Geometry: final body of the model. Coordinates: model frame, mm. A direction names the side the tool comes from. Give positions to 0.01 mm unless a question says otherwise; leave off trailing zeros. Loops run counter-clockwise (first coordinate to the right, second up) from the corner with the lowest first, then second, coordinate; pieces in that order, holes last. Notation, with made-up numbers: (27.5, -9.5) - (79.5, -9.5) arc R19 cw to (79.5, 13.5) - close; hole circle Ø11 at (-15.75, -33.75). An arc over 180 degrees is marked (long way). Answer in a Markdown table with one row per item.
from build123d import *

# Parameters (mm, degrees)
SKETCH1_W           = 114.3
SKETCH1_H           = 177.8
BOSS_EXTRUDE1_DEPTH = 3.9624
CUT_EXTRUDE2_START  = 3.9624
SKETCH2_W           = 184.15
SKETCH2_H           = 53.975
CUT_EXTRUDE2_DEPTH  = 110.721716912
CUT_EXTRUDE4_START  = 3.9624
SKETCH3_R           = 5.1562
CUT_EXTRUDE4_DEPTH  = 110.721716912
CUT_EXTRUDE6_START  = 3.9624
SKETCH4_R           = 5.1562
CUT_EXTRUDE6_DEPTH  = 110.721716912
CUT_EXTRUDE8_START  = 3.9624
SKETCH5_R           = 5.1562
CUT_EXTRUDE8_DEPTH  = 110.721716912
CUT_EXTRUDE10_START = 3.9624
SKETCH6_R           = 2.5781
CUT_EXTRUDE10_DEPTH = 114.3
CUT_EXTRUDE12_START = 3.9624
SKETCH7_R           = 2.5781
CUT_EXTRUDE12_DEPTH = 114.3


with BuildPart() as part:
    # Sketch1 → Boss-Extrude1 (new, symmetric)
    with BuildSketch(Plane(origin=(0, 0, 0), x_dir=(1, 0, 0), z_dir=(0, 1, 0))):
        Rectangle(SKETCH1_W, SKETCH1_H)
    extrude(amount=BOSS_EXTRUDE1_DEPTH, both=True)

    # Sketch2 → Cut-Extrude2 (cut, through all)
    with BuildSketch(Plane(origin=(0, 0, 0), x_dir=(1, 0, 0), z_dir=(0, 1, 0)).offset(CUT_EXTRUDE2_START)):
        with Locations((-79.375, -7.9375)):
            Rectangle(SKETCH2_W, SKETCH2_H)
    extrude(amount=-CUT_EXTRUDE2_DEPTH, mode=Mode.SUBTRACT)

    # Sketch3 → Cut-Extrude4 (cut, through all)
    with BuildSketch(Plane(origin=(0, 0, 0), x_dir=(1, 0, 0), z_dir=(0, 1, 0)).offset(CUT_EXTRUDE4_START)):
        with Locations(Location((-38.1, -79.375, 0), (0, 0, 270))):
            Circle(SKETCH3_R)
        with Locations(Location((-38.1, 79.375, 0), (0, 0, 270))):
            Circle(SKETCH3_R)
    extrude(amount=-CUT_EXTRUDE4_DEPTH, mode=Mode.SUBTRACT)

    # Sketch4 → Cut-Extrude6 (cut, through all)
    with BuildSketch(Plane(origin=(0, 0, 0), x_dir=(1, 0, 0), z_dir=(0, 1, 0)).offset(CUT_EXTRUDE6_START)):
        with Locations(Location((1.5748, -79.375, 0), (0, 0, 270))):
            Circle(SKETCH4_R)
        with Locations(Location((1.5748, 79.375, 0), (0, 0, 270))):
            Circle(SKETCH4_R)
    extrude(amount=-CUT_EXTRUDE6_DEPTH, mode=Mode.SUBTRACT)

    # Sketch5 → Cut-Extrude8 (cut, through all)
    with BuildSketch(Plane(origin=(0, 0, 0), x_dir=(1, 0, 0), z_dir=(0, 1, 0)).offset(CUT_EXTRUDE8_START)):
        with Locations(Location((41.275, -79.375, 0), (0, 0, 270))):
            Circle(SKETCH5_R)
        with Locations(Location((41.275, 79.375, 0), (0, 0, 270))):
            Circle(SKETCH5_R)
    extrude(amount=-CUT_EXTRUDE8_DEPTH, mode=Mode.SUBTRACT)

    # Sketch6 → Cut-Extrude10 (cut)
    with BuildSketch(Plane(origin=(0, 0, 0), x_dir=(1, 0, 0), z_dir=(0, 1, 0)).offset(CUT_EXTRUDE10_START)):
        with Locations(Location((-41.9862, -45.5422, 0), (0, 0, 270))):
            Circle(SKETCH6_R)
        with Locations(Location((-7.0612, -45.5422, 0), (0, 0, 270))):
            Circle(SKETCH6_R)
        with Locations(Location((27.8638, -45.5422, 0), (0, 0, 270))):
            Circle(SKETCH6_R)
        with Locations(Location((-41.9862, 28.8798, 0), (0, 0, 270))):
            Circle(SKETCH6_R)
        with Locations(Location((-7.0612, 28.8798, 0), (0, 0, 270))):
            Circle(SKETCH6_R)
        with Locations(Location((27.8638, 28.8798, 0), (0, 0, 270))):
            Circle(SKETCH6_R)
    extrude(amount=-CUT_EXTRUDE10_DEPTH, mode=Mode.SUBTRACT)

    # Sketch7 → Cut-Extrude12 (cut)
    with BuildSketch(Plane(origin=(0, 0, 0), x_dir=(1, 0, 0), z_dir=(0, 1, 0)).offset(CUT_EXTRUDE12_START)):
        with Locations(Location((27.8638, -8.3312, 0), (0, 0, 270))):
            Circle(SKETCH7_R)
    extrude(amount=-CUT_EXTRUDE12_DEPTH, mode=Mode.SUBTRACT)


solid = part.part
Q1. Cut plane D-D (x = 43). Output: boundary loops of the cut face in (y, z), and give its area (4 significant figures).
Check values:
| item | result |
|---|---|
| outline | (-3.96, -88.9) - (3.96, -88.9) - (3.96, -84.23) - (-3.96, -84.23) - close; (-3.96, -74.52) - (3.96, -74.52) - (3.96, 74.52) - (-3.96, 74.52) - close; (-3.96, 84.23) - (3.96, 84.23) - (3.96, 88.9) - (-3.96, 88.9) - close |
| area | 1,255 mm² |
Q2. First-contact query: pin 1 (4 mm diameter, centred on x = -7.06, z = -28.88, fed in from -Y). Flat tip, straight axial feed; report the tip coordinate or a pass-through.
Check values:
| item | result |
|---|---|
| pin 1 | through |
Q3. Reachability of faces 1 (the flat face through (-1, 3.962, -21)), 2 (the flat face through (12.7, 0, 8)) from +Z, -Z, +X, -X, +Y, -Y: full face, straight path, thin tool, end or side. Return the list, or none.
Check values:
| item | result |
|---|---|
| face 1 | +Z, -Z, +X, -X, +Y |
| face 2 | -X, +Y, -Y |
Q4. Material intervals for line 1 along X through (y, z) = (-1.25, -28.5); line 2 along X through (y, z) = (3, 79.5); line 3 along Z through (x, y) = (-45, -2.5) (3 decimals), sorted ascending.
Check values:
| item | result |
|---|---|
| line 1 | -57.15 to -44.54, -39.44 to -9.61, -4.51 to 25.31, 30.41 to 57.15 |
| line 2 | -57.15 to -43.25, -32.95 to -3.58, 6.73 to 36.12, 46.43 to 57.15 |
| line 3 | -88.9 to -19.05, 34.925 to 88.9 |
Q5. Cut plane A-A (x = -23). Output: boundary loops of the cut face in (y, z) (3 decimals), and give its area (3 significant figures).
Check values:
| item | result |
|---|---|
| outline | (-3.962, -88.9) - (3.962, -88.9) - (3.962, -19.05) - (-3.962, -19.05) - close; (-3.962, 34.925) - (3.962, 34.925) - (3.962, 88.9) - (-3.962, 88.9) - close |
| area | 981 mm² |
Q6. Draft query along Z for faces 3 (the cylindrical face through (25.347, 0.055, 7.772)), 4 (the flat face through (-1, -3.962, -21)). Return one class per face: pulls with the +Z half, pulls with the -Z half, needs draft (parallel to the pull), parting line crosses it, or undercut.
Check values:
| item | result |
|---|---|
| face 3 | undercut |
| face 4 | needs draft |
Q7. Cut plane C-C (y = -1). Give the number of separate pieces and of enclosed holes in the cut face, and give its area (3 significant figures).
Check values:
| item | result |
|---|---|
| separate pieces | 1 |
| enclosed holes | 13 |
| area | 15,900 mm² |
Q8. Cut plane B-B (x = 3.5). Output: boundary loops of the cut face in (y, z) (3 decimals), and give its area (3 significant figures).
Check values:
| item | result |
|---|---|
| outline | (-3.962, -88.9) - (3.962, -88.9) - (3.962, -84.158) - (-3.962, -84.158) - close; (-3.962, -74.592) - (3.962, -74.592) - (3.962, -19.05) - (-3.962, -19.05) - close; (-3.962, 34.925) - (3.962, 34.925) - (3.962, 74.592) - (-3.962, 74.592) - close; (-3.962, 84.158) - (3.962, 84.158) - (3.962, 88.9) - (-3.962, 88.9) - close |
| area | 830 mm² |
